from build123d import *

# Parameters (mm, degrees)
SKETCH1_R           = 75
BOSS_EXTRUDE1_DEPTH = 20
BOSS_EXTRUDE1_TAPER = 7
SKETCH6_R           = 25
SKETCH6_R_2         = 3.4
CUT_EXTRUDE1_DEPTH  = 21


with BuildPart() as part:
    # Sketch1 → Boss-Extrude1 (new body)
    with BuildSketch(Plane.XY):
        Circle(SKETCH1_R)
    extrude(amount=BOSS_EXTRUDE1_DEPTH, taper=BOSS_EXTRUDE1_TAPER)

    # Sketch6 → Cut-Extrude1 (cut, through all)
    with BuildSketch(Plane(origin=(0, 0, 0), x_dir=(-1, 0, 0), z_dir=(0, 0, -1))):
        Circle(SKETCH6_R)
        with Locations((0, 50)):
            Circle(SKETCH6_R_2)
        with Locations((50, 0)):
            Circle(SKETCH6_R_2)
        with Locations((0, -50)):
            Circle(SKETCH6_R_2)
        with Locations((-50, 0)):
            Circle(SKETCH6_R_2)
    extrude(amount=-CUT_EXTRUDE1_DEPTH, mode=Mode.SUBTRACT)


solid = part.part
CAD build for the part. Positions are in the model's coordinates, mm. Give positions to 0.01 mm unless a question says otherwise; leave off trailing zeros. Write each loop counter-clockwise with the first axis right and the second up, starting at its lowest first coordinate (ties: lowest second). Pieces come first, ordered by that corner, then holes. Notation, with made-up numbers: (8.25, -14) - (60.25, -14) arc R25 cw to (60.25, 7) - close; hole circle Ø3 at (10.25, 88.5). An arc over 180 degrees is marked (long way). Put each result on its own line as item: value.
(1) Pull direction X, two halves, no side cores. Call faces 1 (the conical face through (39.06, 61.27, 19.03)), 2 (the cylindrical face through (0.44, 53.37, 9.86)), 3 (the flat face through (31, 1, 20)): released by +X, released by -X, zero draft, split by the parting line, or undercut.
Working result:
face 1: split by the parting line
face 2: undercut
face 3: zero draft
(2) Saw through at C-C (z = 13.5). List the corners of the cut face in (x, y), then the cut area to 3 significant figures.
Working result:
outline: circle Ø146.68 at (0, 0); hole circle Ø6.8 at (-50, 0); hole circle Ø50 at (0, 0); hole circle Ø6.8 at (0, -50); hole circle Ø6.8 at (0, 50); hole circle Ø6.8 at (50, 0)
area: 14,800 mm^2
(3) Drop flat-ended pins along their axis: pin 1 Ø2 at (x, y) = (5, 44.5) entering from -Z; pin 2 Ø2 at (y, z) = (-45.5, 17.5) entering from +X; pin 3 Ø1 at (x, z) = (46.5, 6.5) entering from +Y; pin 4 Ø4 at (x, z) = (-34.5, 3.5) entering from -Y. Give the stop position or say it passes through.
Working result:
pin 1: z = 0
pin 2: x = 57.7
pin 3: y = 58.23
pin 4: y = -67.15
(4) Wall check: L1, parallel to Y at x = -2, z = 6.5; L2, parallel to Y at x = 0, z = 15.25; L3, parallel to Y at x = -50, z = 11.5. Give the ranges that are in metal, low to high.
Working result:
L1: -74.17 to -52.75, -47.25 to -24.92, 24.92 to 47.25, 52.75 to 74.17
L2: -73.13 to -53.4, -46.6 to -25, 25 to 46.6, 53.4 to 73.13
L3: -53.99 to -3.4, 3.4 to 53.99
(5) Saw through at A-A (x = 0). List the corners of the cut face in (y, z).
Working result:
outline: (-75, 0) - (-53.4, 0) - (-53.4, 20) - (-72.54, 20) - close; (-46.6, 0) - (-25, 0) - (-25, 20) - (-46.6, 20) - close; (25, 0) - (46.6, 0) - (46.6, 20) - (25, 20) - close; (53.4, 0) - (75, 0) - (72.54, 20) - (53.4, 20) - close
(6) Saw through at D-D (z = 2.75). List the corners of the cut face in (x, y).
Working result:
outline: circle Ø149.32 at (0, 0); hole circle Ø6.8 at (-50, 0); hole circle Ø50 at (0, 0); hole circle Ø6.8 at (0, -50); hole circle Ø6.8 at (0, 50); hole circle Ø6.8 at (50, 0)
